Autodesk Fusion 360 part; units mm, degrees
sketch "Sketch1" plane through (0, 0, 0) normal (0, 0, 1) x (1, 0, 0)
  line L0 (0.0707, 5.374) -> (5.374, 0.0707)
  line L1 (5.374, 0.0707) -> (5.2326, -0.0707)
  line L2 (5.2326, -0.0707) -> (-0.0707, 5.2326)
  line L3 (-0.0707, 5.2326) -> (0.0707, 5.374)
  line L4 (0, 0) -> (25, 0) construction
  line L5 (0.0707, -5.374) -> (5.374, -0.0707)
  line L6 (-0.0707, -5.2326) -> (0.0707, -5.374)
  line L7 (5.2326, 0.0707) -> (-0.0707, -5.2326)
  line L8 (5.374, -0.0707) -> (5.2326, 0.0707)
  line L9 (5.1619, 0.2) -> (15, 0.2)
  line L10 (15, 0.2) -> (15, -0.2)
  line L11 (15, -0.2) -> (5.1619, -0.2)
  line L12 (5.1619, -0.2) -> (5.1619, 0.2)
  line L13 (0, -5.3033) -> (0, 5.3033) construction
  point P0 (0, 5.3033)
  point P1 (0, -5.3033)
  point P2 (5.3033, 0)
  point P3 (5.1619, 0)
  dimension "d39" = 25
  dimension "d40" = 0.2
  dimension "d41" = 45
  dimension "d42" = 0.4
  dimension "d46" = 15
  dimension "d48" = 7.5
extrude "Extrude1" add sketch "Sketch1" along normal blind 0.2
equation "d1001 = depth"
equation "channelwidth = 0.2 mm"
equation "depth = 0.2 mm"
equation "length = 15 mm"
equation "d40 = channelwidth"
equation "d41 = angle"
equation "d42 = channelwidth * 2"
equation "angle = 45 deg"
equation "d46 = length"
equation "d48 = length / 2"
equation "combinedwidth = channelwidth * 2"
Geometry check sheet. Reference: the model listing, model coordinates, mm. Give positions to 0.01 mm unless a question says otherwise; leave off trailing zeros. Order: outer loops, then holes, each group sorted by start corner. A loop starts at its lowest first (then second) coordinate and runs counter-clockwise, first axis right, second up.
1) Cross-section at B-B (x = 2). Record the boundary of the cut face in (y, z).
Results are:
outline: (-3.44, 0) - (-3.16, 0) - (-3.16, 0.2) - (-3.44, 0.2) - close; (3.16, 0) - (3.44, 0) - (3.44, 0.2) - (3.16, 0.2) - close
2) Cross-section at C-C (x = 10.25). Record the boundary of the cut face in (y, z).
Results are:
outline: (-0.2, 0) - (0.2, 0) - (0.2, 0.2) - (-0.2, 0.2) - close
3) Cross-section at D-D (y = -2.75). Record the boundary of the cut face in (x, z).
Results are:
outline: (2.41, 0) - (2.69, 0) - (2.69, 0.2) - (2.41, 0.2) - close
4) Cross-section at A-A (z = 0.1). Record the boundary of the cut face in (x, y).
Results are:
outline: (-0.07, -5.23) - (0.07, -5.37) - (5.24, -0.2) - (15, -0.2) - (15, 0.2) - (5.24, 0.2) - (0.07, 5.37) - (-0.07, 5.23) - (5.16, 0) - close
5) Material ranges on probe 1 along Y at (x, z) = (10.75, 0.15); probe 2 along Y at (x, z) = (2.75, 0.15); probe 3 along Y at (x, z) = (4.25, 0.05), recorded low to high.
Results are:
probe 1: y = -0.2 to 0.2
probe 2: y = -2.69 to -2.41, 2.41 to 2.69
probe 3: y = -1.19 to -0.91, 0.91 to 1.19
